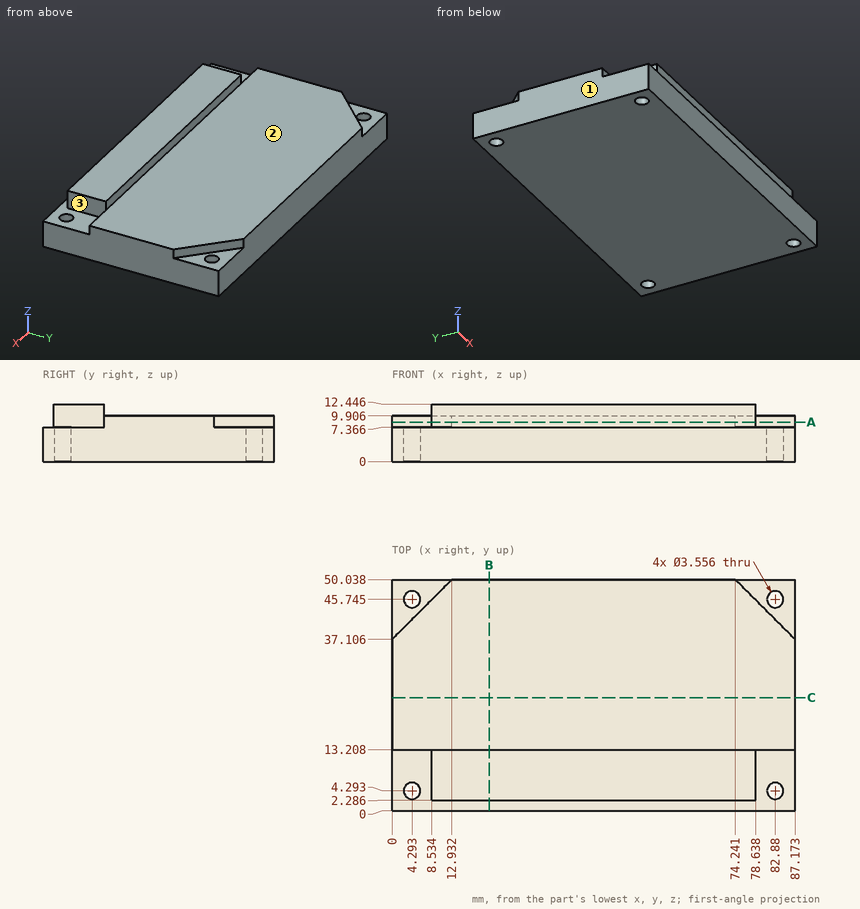
Study the drawing (mm; zero at the part's minimum x, y, z) and answer. A direction names the side the tool comes from. Coordinates: 2 decimals unless noted, no trailing zeros. Write each loop counter-clockwise with the first axis right and the second up, starting at its lowest first coordinate (ties: lowest second). Pieces come first, ordered by that corner, then holes. Notation, with made-up numbers: (89.5, 12.25) -> (109.5, 12.25) arc R19 cw to (109.5, 46.25) -> close; hole circle Ø3 at (-0.75, 89.25). An arc over 180 degrees is marked (long way). Write each question's results on one line, items separated by ' | '. Start each with the question number.
1) Flat-ended cylindrical pins translate along their axes: pin 1 Ø4 at (y, z) = (9, 10) entering from -X; pin 2 Ø4 at (y, z) = (7, 10.5) entering from +X; pin 3 Ø1 at (x, z) = (71, 8.5) entering from -Y. Find the tip coordinate at first contact, or state that the pin passes through.
2) A tool of negligible diameter and unlimited length cuts with its end or side. For the marked faces 1, 2 and 3, from which of +Z, -Z, +X, -X, +Y, -Y can it reach the whole face along a straight path? Write none if from no direction.
3) A cutting plane is placed at C-C (y = 24.5). Determine the outline of the cut face in (x, z).
4) A cutting plane is placed at B-B (x = 21). Determine the outline of the cut face in (y, z).
5) A cutting plane is placed at A-A (z = 8.5). Determine the outline of the cut face in (x, y) (1 decimal), then the cut area to 3 significant figures.
6) Straight lines are drawn through the part: probe 1 along Y at (x, z) = (82, 2); probe 2 along Z at (x, y) = (34, 16.5); probe 3 along X at (y, z) = (5.5, 2) (1 decimal). For each, find the intervals that lie inside material, in ascending order.
Values follow:
1) pin 1: x = 8.53 | pin 2: x = 78.64 | pin 3: y = 2.29
2) face 1: +Z, -Z, -X, +Y, -Y | face 2: +Z, +X, -X, +Y | face 3: +Z, +X, -Y
3) outline: (0, 0) -> (87.17, 0) -> (87.17, 9.91) -> (0, 9.91) -> close
4) outline: (0, 0) -> (50.04, 0) -> (50.04, 9.91) -> (13.21, 9.91) -> (13.21, 12.45) -> (2.29, 12.45) -> (2.29, 7.37) -> (0, 7.37) -> close
5) outline: (0, 13.2) -> (8.5, 13.2) -> (8.5, 2.3) -> (78.6, 2.3) -> (78.6, 13.2) -> (87.2, 13.2) -> (87.2, 37.1) -> (74.2, 50) -> (12.9, 50) -> (0, 37.1) -> close | area: 3,810 mm²
6) probe 1: 0 to 2.75, 5.84 to 44.2, 47.29 to 50.04 | probe 2: 0 to 9.91 | probe 3: 0 to 3, 5.6 to 81.6, 84.2 to 87.2
